Source: CAD feature listing. Evaluate the final solid. Frame: model axes, mm. A direction names the side the tool comes from. Round coordinates to 2 decimals unless told otherwise and drop trailing zeros. Order: outer loops, then holes, each group sorted by start corner. A loop starts at its lowest first (then second) coordinate and runs counter-clockwise, first axis right, second up. Notation, with made-up numbers: (-4, -20) - (2, -20) arc R25 cw to (2, 13) - close; hole circle Ø11 at (61, 17). An arc over 180 degrees is marked (long way). Return JSON: item names as keys, results as strings. Group by question number.
1) Ray query, line 1 (Y direction, x = -7.35, z = 0); line 2 (Z direction, x = -0.5, y = -3.25) (3 decimals); line 3 (X direction, y = 11.5, z = -2). Return the intervals inside material, ascending. Write a range as from..to.
2) Mould query, pull axis Z, two halves, no side actions, for faces 1 (the flat face through (3.5, 11, 0)), 2 (the flat face through (0, -2, -7.5)), 3 (the flat face through (0, 2, -6)). Classes: pulls with the +Z half, pulls with the -Z half, needs draft (parallel to the pull), parting line crosses it, or undercut.
3) Section A-A, the plane x = 0. Return loops of the section in (y, z) (3 decimals).
4) Access query for faces 4 (the flat face through (0, 16, 8)), 5 (the flat face through (9, 8, 4)), 6 (the flat face through (0, 9, -5.4)), 7 (the flat face through (0, 0, 0)), 8 (the flat face through (-3.5, 11, 0)). Directions: +Z, -Z, +X, -X, +Y, -Y. A direction counts if a zero-diameter tool reaches every point of the face in a straight line with its end or side. Return the directions, or none.
5) Section D-D, the plane x = -4.75. Return loops of the section in (y, z) (3 decimals), plus the area to 3 significant figures.
6) Section B-B, the plane z = 17.5. Return loops of the section in (x, y).
7) Section C-C, the plane y = 13.25. Return loops of the section in (x, z).
8) Contact query for flat-ended pins moving along their axis: P1, Ø3, axis at x = 5, y = 8.5, coming from the +Z side; P2, Ø4, axis at x = -6, y = 10, coming from the +Z side; P3, Ø0.6, axis at x = -3, z = -6.5, coming from the +Y side; P4, Ø1.8, axis at x = -4.5, y = 12.5, coming from the -Z side. Output: stop coordinate, or through.
```python
from build123d import *

# Parameters (mm, degrees)
IZIM1_W                     = 18
IZIM1_H                     = 15
Y_KSEKLIK_EKSTR_ZYON1_DEPTH = 16
IZIM4_R                     = 2
KES_EKSTR_ZYON3_DEPTH       = 26.223996511
IZIM5_W                     = 3.5
IZIM5_H                     = 7.2
KES_EKSTR_ZYON4_DEPTH       = 9
KES_EKSTR_ZYON6_DEPTH       = 1.75
KES_EKSTR_ZYON14_DEPTH      = 1.75
IZIM11_W                    = 18
IZIM11_H                    = 5
MAKAS_DELI_I_DEPTH          = 14
IZIM12_R                    = 1.65
KES_EKSTR_ZYON10_DEPTH      = 8
PAH1_SIZE                   = 11
PAH1_SIZE_2                 = 3
IZIM15_W                    = 18
IZIM15_H                    = 15
ALT_SLOT_DEPTH              = 6
IZIM16_W                    = 10.15
IZIM16_H                    = 4.15
IZIM16_W_2                  = 2.1
IZIM16_H_2                  = 14
KES_EKSTR_ZYON15_DEPTH      = 33.283896915


with BuildPart() as part:
    # Çizim1 → Yükseklik-Ekstrüzyon1 (new body)
    with BuildSketch(Plane(origin=(0, 0, 0), x_dir=(1, 0, 0), z_dir=(0, 1, 0))):
        Rectangle(IZIM1_W, IZIM1_H)
    extrude(amount=Y_KSEKLIK_EKSTR_ZYON1_DEPTH)

    # Çizim4 → Kes-Ekstrüzyon3 (cut, through all)
    with BuildSketch(Plane.ZY.offset(9)):
        with Locations((0, 7)):
            Circle(IZIM4_R)
    extrude(amount=-KES_EKSTR_ZYON3_DEPTH, mode=Mode.SUBTRACT)

    # Çizim5 → Kes-Ekstrüzyon4 (cut)
    with BuildSketch(Plane(origin=(0, 16, 0), x_dir=(1, 0, 0), z_dir=(0, 1, 0))):
        with Locations((5.25, 0)):
            Rectangle(IZIM5_W, IZIM5_H)
        with Locations((-5.25, 0)):
            Rectangle(IZIM5_W, IZIM5_H)
    extrude(amount=-KES_EKSTR_ZYON4_DEPTH, mode=Mode.SUBTRACT)

    # Çizim6 → Kes-Ekstrüzyon6 (cut, symmetric)
    with BuildSketch(Plane.ZY.offset(-5.25)):
        Polygon((3.6, 9.078460969), (0, 11.156921938), (-3.6, 9.078460969), (-3.6, 4.921539031), (0, 2.843078062), (3.6, 4.921539031), align=None)
    extrude(amount=KES_EKSTR_ZYON6_DEPTH, both=True, mode=Mode.SUBTRACT)

    # Çizim14 → Kes-Ekstrüzyon14 (cut, symmetric)
    with BuildSketch(Plane.ZY.offset(5.25)):
        Polygon((3.6, 9.078460969), (0, 11.156921938), (-3.6, 9.078460969), (-3.6, 4.921539031), (0, 2.843078062), (3.6, 4.921539031), align=None)
    extrude(amount=KES_EKSTR_ZYON14_DEPTH, both=True, mode=Mode.SUBTRACT)

    # Çizim11 → makas deliği (add)
    with BuildSketch(Plane(origin=(0, 0, 7.5), x_dir=(-1, 0, 0), z_dir=(0, 0, -1))):
        with Locations((0, 13.5)):
            Rectangle(IZIM11_W, IZIM11_H)
    extrude(amount=-MAKAS_DELI_I_DEPTH)

    # Çizim12 → Kes-Ekstrüzyon10 (cut)
    with BuildSketch(Plane(origin=(0, 16, 0), x_dir=(1, 0, 0), z_dir=(0, 1, 0))):
        with Locations(Location((0, -17.5, 0), (0, 0, 270))):
            Circle(IZIM12_R)
    extrude(amount=-KES_EKSTR_ZYON10_DEPTH, mode=Mode.SUBTRACT)

    # Pah1
    # the kernel refuses this chamfer: 11, 3 mm, written as the material it adds along each edge
    with BuildSketch(Plane(origin=(9, 11, 7.5), x_dir=(0, -0.9999486586881362, -0.010133113430599267), z_dir=(-1, 0, 0))) as pah1_piece_1_section:
        Polygon((PAH1_SIZE * 0.999948658688, PAH1_SIZE * 0.0101331134306), (-PAH1_SIZE_2 * 0.0101331134306, PAH1_SIZE_2 * 0.999948658688), (0, 0), align=None)
    pah1_piece_1 = extrude(amount=18, mode=Mode.PRIVATE)
    pah1_piece_1 = split(pah1_piece_1, bisect_by=Plane(origin=(0, 0, 8.392972415), z_dir=(0, 1, 0)), keep=Keep.TOP, mode=Mode.PRIVATE)
    add(pah1_piece_1)

    # Çizim15 → alt slot (add)
    with BuildSketch(Plane.XZ):
        Rectangle(IZIM15_W, IZIM15_H)
    extrude(amount=ALT_SLOT_DEPTH)

    # Çizim16 → Kes-Ekstrüzyon15 (cut, through all)
    with BuildSketch(Plane.ZY.offset(9)):
        with Locations((0, -2.075)):
            Rectangle(IZIM16_W, IZIM16_H)
        with Locations((-6.45, 9)):
            Rectangle(IZIM16_W_2, IZIM16_H_2)
    extrude(amount=-KES_EKSTR_ZYON15_DEPTH, mode=Mode.SUBTRACT)


solid = part.part
```
Geometry check:
{
 "1": {"line 1": "-6..-4.15, 0..5, 9..16", "line 2": "-7.5..-5.075, 5.075..7.5", "line 3": "-9..-7, -3.5..3.5, 7..9"},
 "2": {"face 1": "undercut", "face 2": "pulls with the -Z half", "face 3": "needs draft"},
 "3": {"outline": "(-6, -7.5) - (2, -7.5) - (2, -5.4) - (16, -5.4) - (16, 15.85) - (11, 15.85) - (11, 10.5) - (0, 7.5) - (-6, 7.5) - close; (11, 19.15) - (16, 19.15) - (16, 21.5) - (11, 21.5) - close; hole (-4.15, -5.075) - (0, -5.075) - (0, 5.075) - (-4.15, 5.075) - close; hole circle Ø4 at (7, 0)"},
 "4": {"face 4": "+Z, -Z, +X, -X, +Y", "face 5": "+Z, -Z, +X, +Y, -Y", "face 6": "-Z, +X, -X, +Y", "face 7": "+X, -X", "face 8": "+Y"},
 "5": {"outline": "(-6, -7.5) - (2, -7.5) - (2, -5.4) - (16, -5.4) - (16, -3.6) - (4.922, -3.6) - (2.843, 0) - (4.922, 3.6) - (16, 3.6) - (16, 21.5) - (11, 21.5) - (11, 10.5) - (0, 7.5) - (-6, 7.5) - close; hole (-4.15, -5.075) - (0, -5.075) - (0, 5.075) - (-4.15, 5.075) - close", "area": "258 mm2"},
 "6": {"outline": "(-9, 11) - (-1.65, 11) - (-1.65, 16) - (-9, 16) - close; (1.65, 11) - (9, 11) - (9, 16) - (1.65, 16) - close"},
 "7": {"outline": "(-9, -5.4) - (9, -5.4) - (9, 21.5) - (-9, 21.5) - close; hole (-7, -3.6) - (-3.5, -3.6) - (-3.5, 3.6) - (-7, 3.6) - close; hole circle Ø3.3 at (0, 17.5); hole (3.5, -3.6) - (7, -3.6) - (7, 3.6) - (3.5, 3.6) - close"},
 "8": {"P1": "z = 10.23", "P2": "z = 21.5", "P3": "y = 2", "P4": "z = -5.4"}
}
